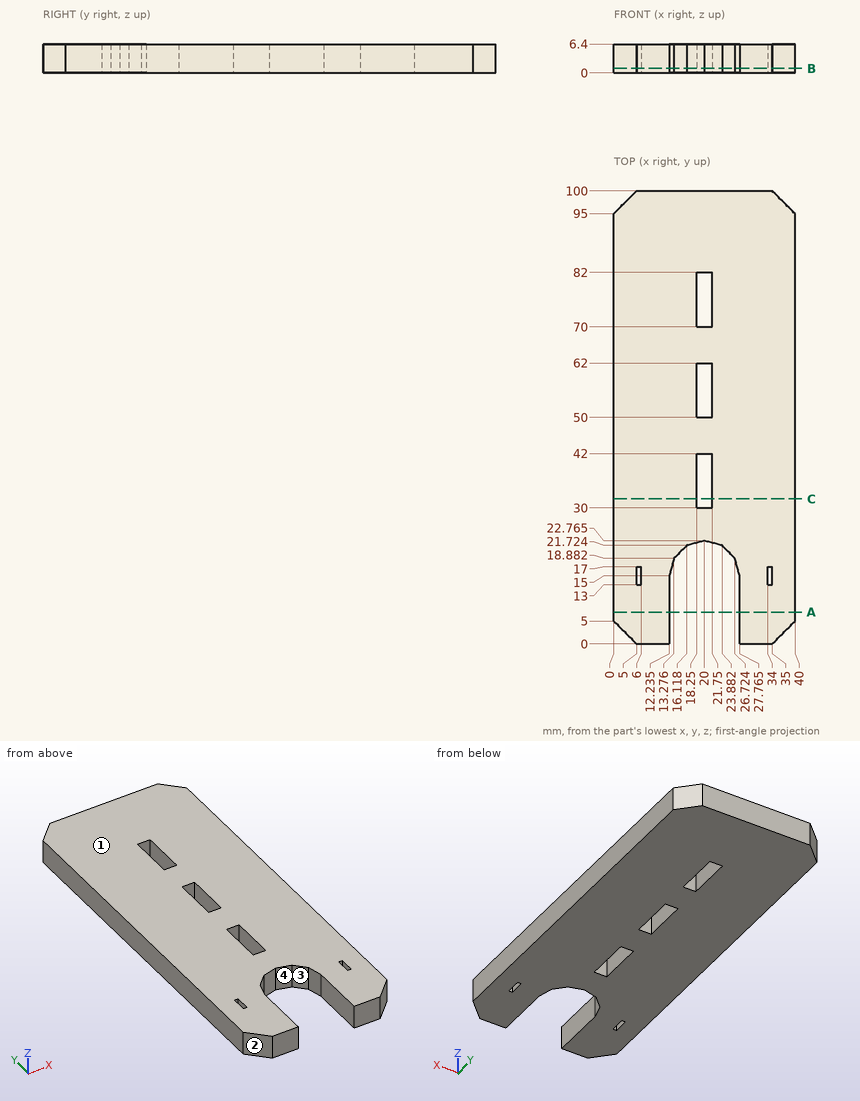
Part print with two shaded views. Sizes in mm from the minimum x, y, z corner. Round coordinates to 2 decimals unless told otherwise and drop trailing zeros. Loops run counter-clockwise (first coordinate to the right, second up) from the corner with the lowest first, then second, coordinate; pieces in that order, holes last. Notation, with made-up numbers: (52, 51) - (78, 51) arc R23 ccw to (78, 86) - close; hole circle Ø1 at (71, 41.25). An arc over 180 degrees is marked (long way). Put each result on its own line as item: value.
1. Wall check: line 1 (X direction, y = 40.5, z = 2); line 2 (Y direction, x = 21.5, z = 2); line 3 (X direction, y = 15, z = 4.5) (1 decimal). Give the ranges that are in metal, low to high.
Geometry check:
line 1: 0 to 18.25, 21.75 to 40
line 2: 22.36 to 30, 42 to 50, 62 to 70, 82 to 100
line 3: 0 to 5, 6 to 12.2, 27.8 to 34, 35 to 40
2. Slice it at B-B on z = 1. Give the number of separate pieces and of enclosed holes in the cut face, and give its area (3 significant figures).
Geometry check:
separate pieces: 1
enclosed holes: 5
area: 3,490 mm²
3. Two-plate mould, pull along X, no slides. Class the marked faces 1, 2, 3 and 4: released by +X, released by -X, zero draft, split by the parting line, or undercut.
Geometry check:
face 1: zero draft
face 2: released by -X
face 3: undercut
face 4: undercut
4. Slice it at C-C on y = 32. List the corners of the cut face in (x, z).
Geometry check:
outline: (0, 0) - (18.25, 0) - (18.25, 6.4) - (0, 6.4) - close; (21.75, 0) - (40, 0) - (40, 6.4) - (21.75, 6.4) - close
5. Slice it at A-A on y = 7. List the corners of the cut face in (x, z) (1 decimal).
Geometry check:
outline: (0, 0) - (12.2, 0) - (12.2, 6.4) - (0, 6.4) - close; (27.8, 0) - (40, 0) - (40, 6.4) - (27.8, 6.4) - close
6. Pin check, flat tips, straight feed: P1, Ø6, axis at x = 9.5, y = 11.5, coming from the -Z side; P2, Ø3, axis at x = 20.5, z = 4, coming from the -Y side. Stop position of each tip, or through.
Geometry check:
P1: z = 0
P2: y = 22.23
